Verification items for the finished model (mm, model axes). A direction names the side the tool comes from. Round coordinates to 2 decimals unless told otherwise and drop trailing zeros. Use CSV: the item, a comma, the result in double quotes.
```python
from build123d import *

# Parameters (mm, degrees)
F5_DEPTH       = 40
F10_DEPTH      = 100
F10_DEPTH_BACK = 100
F12_DEPTH      = 100
F12_DEPTH_BACK = 25


with BuildPart() as f3:
    # F0 (on Top) → F3 section 0
    with BuildSketch(Plane.XY):
        Polygon((49.7695431113, -86.2033773383), (49.7695431113, 86.2033773383), (-99.5390862226, 0), align=None)
    # F2 (on offset) → F3 section 1
    with BuildSketch(Plane.XY.offset(120)):
        Polygon((19.951004535, -34.5561535166), (19.951004535, 34.5561535166), (-39.9020090699, 0), align=None)
    loft()

    # F4 (on face) → F5 (cut)
    with BuildSketch(Plane.XY.offset(120)):
        Polygon((4.6946327202, -25.7478831425), (4.6946327202, 25.7478831425), (-4.6946327202, 20.326988213), (-4.6946327202, -20.326988213), align=None)
        Polygon((4.6946327202, 25.7478831425), (4.6946327202, 48.1600351632), (-4.6946327202, 48.1600351632), (-4.6946327202, 20.326988213), align=None)
        Polygon((4.6946327202, -48.1600351632), (4.6946327202, -25.7478831425), (-4.6946327202, -20.326988213), (-4.6946327202, -48.1600351632), align=None)
    extrude(amount=-F5_DEPTH, mode=Mode.SUBTRACT)

    # F8: sweep along a path in F7
    with BuildLine(Plane.XZ) as f8_path:
        Line((-31.9719016552, 120.4966977239), (-107.2546765208, 0))
    # F6 (on face) → F8 (sweep, cut)
    with BuildSketch(Plane.XY.offset(120)):
        Polygon((-40.3947457671, 19.6701809764), (-40.3947457671, -19.6701809764), (-24.4082733989, -19.6701809764), (-24.4082733989, -8.9453124604), (-24.4082733989, 19.6701809764), align=None)
    sweep(path=f8_path.line, mode=Mode.SUBTRACT)

    # F9 (on Front) → F10 (cut, two sides)
    with BuildSketch(Plane.XZ) as f10_sk:
        Polygon((-75.3909720121, 6.0918268561), (28.532076442, 6.0918268561), (-23.429447785, 96.0918268561), align=None)
    extrude(amount=-F10_DEPTH, mode=Mode.SUBTRACT)
    extrude(f10_sk.sketch, amount=F10_DEPTH_BACK, mode=Mode.SUBTRACT)

    # F11 (on Right) → F12 (cut, two sides)
    with BuildSketch(Plane.YZ) as f12_sk:
        Polygon((-51.9615242271, 6.0918268561), (51.9615242271, 6.0918268561), (0, 96.0918268561), align=None)
    extrude(amount=F12_DEPTH, mode=Mode.SUBTRACT)
    extrude(f12_sk.sketch, amount=-F12_DEPTH_BACK, mode=Mode.SUBTRACT)


solid = f3.part
```
Q1. Mould release check, pull along X, two halves, no side actions. Record for faces 3 (the flat face through (4.597, -33.592, 47.548)), 4 (the flat face through (-54.09, -0.13, 72.49)), 5 (the flat face through (-12, 0, 120)): released by +X, released by -X, zero draft, split by the parting line, or undercut.
Filled in:
face 3,"undercut"
face 4,"released by -X"
face 5,"zero draft"
Q2. Access from +Z, -Z, +X, -X, +Y, -Y to the whole of each face (thin tool, end or side, straight path). Record for faces 1 (the flat face through (12, 0, 120)), 2 (the flat face through (-4.695, 0, 100)).
Filled in:
face 1,"+Z, +X, -X, +Y, -Y"
face 2,"+Z, +Y, -Y"
Q3. Go/stop test with flat-tipped pins: P1, Ø8, axis at x = -41.5, y = -6.5, coming from the +Z side; P2, Ø6, axis at y = -2, z = 76, coming from the +X side; P3, Ø0.8, axis at y = 0, z = 95, coming from the +X side. Record where each tip stops, or that it passes through.
Filled in:
P1,"z = 99.05"
P2,"x = -33.3"
P3,"x = -25"
Q4. Material ranges on L1, parallel to Z at x = -16, y = -40; L2, parallel to Y at x = -4.5, z = 71; L3, parallel to Z at x = -27.5, y = -3, recorded low to high.
Filled in:
L1,"0 to 6.09"
L2,"-34.5 to -14.49, 14.49 to 34.5"
L3,"0 to 6.09, 89.04 to 115.05"
Q5. Section check A-A (z = 24). State how many separate pieces and enclosed holes the cut face has, plus the area to 3 significant figures.
Filled in:
separate pieces,"3"
enclosed holes,"0"
area,"1,660 mm²"
